Here's how the part is built. I have some questions about the finished solid (model axes, mm). A direction names the side the tool comes from. Coordinates: 2 decimals unless noted, no trailing zeros. Write each loop counter-clockwise with the first axis right and the second up, starting at its lowest first coordinate (ties: lowest second). Pieces come first, ordered by that corner, then holes. Notation, with made-up numbers: M 43.5,78 L 62.5,78 A28 cw 62.5,106 Z; hole C 71,37 d6. An arc over 180 degrees is marked long. Use a Markdown table: item, result.
```python
from build123d import *

# Parameters (mm, degrees)
F1_R     = 15
F2_DEPTH = 10
F0_R     = 9.25
F3_DEPTH = 5
F4_R     = 12.5
F5_DEPTH = 25


with BuildPart() as f2:
    # F1 (on Right) → F2 (new body)
    with BuildSketch(Plane.YZ):
        Circle(F1_R)
    extrude(amount=-F2_DEPTH)

    # F0 (on Right) → F3 (cut)
    with BuildSketch(Plane.YZ):
        Circle(F0_R)
    extrude(amount=-F3_DEPTH, mode=Mode.SUBTRACT)

    # F4 (on face) → F5 (cut)
    with BuildSketch(Plane.YZ.offset(-5)):
        Circle(F4_R)
    extrude(amount=-F5_DEPTH, mode=Mode.SUBTRACT)


solid = f2.part
```
1. Which directions (+Z, -Z, +X, -X, +Y, -Y) give clear straight access to the entire face, cutting with the end or side of a thin tool? Please do faces 4 (the face through (-7.465, 11.923, 3.755)), 5 (the face through (-10, -3.4, 12.3)).
Answers follow:
| item | result |
|---|---|
| face 4 | -X |
| face 5 | +Z, -Z, -X, +Y, -Y |
2. Suppose I cut it at D-D on z = -11.25. Write out the boundary of the cut face in (x, y).
Answers follow:
| item | result |
|---|---|
| outline | M -10,-9.92 L 0,-9.92 L 0,9.92 L -10,9.92 L -10,5.45 L -5,5.45 L -5,-5.45 L -10,-5.45 Z |
3. Will these pins go through, and if not, where does the flat tip stop? pin 1 Ø6 at (x, y) = (-1.5, -9.5) entering from +Z; pin 2 Ø1 at (x, z) = (-2, -11.5) entering from +Y; pin 3 Ø6 at (x, z) = (-2.5, 11.5) entering from -Y.
Answers follow:
| item | result |
|---|---|
| pin 1 | stops at z = 13.52 |
| pin 2 | stops at y = 10.2 |
| pin 3 | stops at y = -12.36 |
4. Suppose I cut it at A-A on y = 0. Write out the boundary of the cut face in (x, z), and give its area (3 significant figures).
Answers follow:
| item | result |
|---|---|
| outline | M -10,-15 L 0,-15 L 0,-9.25 L -5,-9.25 L -5,-12.5 L -10,-12.5 Z; M -10,12.5 L -5,12.5 L -5,9.25 L 0,9.25 L 0,15 L -10,15 Z |
| area | 82.5 mm2 |
5. I need wall thicknesses on probe 1 along Z at (x, y) = (-2.8, 0); probe 2 along Z at (x, y) = (-8.5, 0); probe 3 along Y at (x, z) = (-8, -10). Which ranges of each line are inside material? Lowest first, please.
Answers follow:
| item | result |
|---|---|
| probe 1 | z = -15 to -9.25, 9.25 to 15 |
| probe 2 | z = -15 to -12.5, 12.5 to 15 |
| probe 3 | y = -11.18 to -7.5, 7.5 to 11.18 |
6. We'd pull the mould along Y, two halves only. Please class faces 1 (the face through (0, 6.5, 6.9)), 2 (the face through (-2.46, -2.01, -9.03)), 3 (the face through (-4.93, -14.985, 0.66)): +Y half, -Y half, draft (parallel to the pull), parting line (faces both ways), or undercut.
Answers follow:
| item | result |
|---|---|
| face 1 | draft |
| face 2 | undercut |
| face 3 | parting line |
7. Suppose I cut it at C-C on y = -11. Write out the boundary of the cut face in (x, z), and give its area (3 significant figures).
Answers follow:
| item | result |
|---|---|
| outline | M -10,-10.2 L 0,-10.2 L 0,10.2 L -10,10.2 L -10,5.94 L -5,5.94 L -5,-5.94 L -10,-5.94 Z |
| area | 145 mm2 |
